from build123d import *

# Parameters (mm, degrees)
F1_DEPTH = 25.4
F2_W     = 190.5
F2_H     = 12.7
F2_W_2   = 19.05
F3_DEPTH = 254
F4_DEPTH = 25.4


with BuildPart() as f1:
    # F0 (on Top) → F1 (new body)
    with BuildSketch(Plane.XY):
        Polygon((170.6390685204, 0), (-165.9109314796, 0), (-165.9109314796, -161.925), (-153.2109314796, -161.925), (-153.2109314796, -25.4), (157.9390685204, -25.4), (157.9390685204, -161.925), (170.6390685204, -161.925), align=None)
    extrude(amount=F1_DEPTH)

    # F2 (on face) → F3 (join)
    with BuildSketch(Plane.XY.offset(25.4)):
        with Locations((2.3640685204, -19.05)):
            Rectangle(F2_W, F2_H)
        with Locations((2.3640685204, -6.35)):
            Rectangle(F2_W, F2_H)
        with Locations((-102.4109314796, -6.35)):
            Rectangle(F2_W_2, F2_H)
        with Locations((107.1390685204, -6.35)):
            Rectangle(F2_W_2, F2_H)
    extrude(amount=F3_DEPTH)

    # F2 (on face) → F4 (cut)
    with BuildSketch(Plane.XY.offset(25.4)):
        Polygon((116.6640685204, -12.7), (97.6140685204, -12.7), (97.6140685204, -25.4), (157.9390685204, -25.4), (157.9390685204, -12.7), align=None)
        Polygon((-92.8859314796, -25.4), (-92.8859314796, -12.7), (-111.9359314796, -12.7), (-153.2109314796, -12.7), (-153.2109314796, -25.4), align=None)
    extrude(amount=-F4_DEPTH, mode=Mode.SUBTRACT)


solid = f1.part
The model under review builds one solid part; all positions refer to its coordinate system, in mm. A direction names the side the tool comes from. Round coordinates to 2 decimals unless told otherwise and drop trailing zeros. Write each loop counter-clockwise with the first axis right and the second up, starting at its lowest first coordinate (ties: lowest second). Pieces come first, ordered by that corner, then holes. Notation, with made-up numbers: M -1,6.5 L 44,6.5 A25 cw 44,24.5 Z; hole C 20.25,16.25 d4. An arc over 180 degrees is marked long. Use a Markdown table: item, result. Add a question column.
Q1. We need section A-A, the plane y = -54. State the section outline as (x, z) points.
Q2. Machinability: for faces 4 (the face through (-111.936, -6, 151)), 5 (the face through (116.664, -6, 151)), 6 (the face through (115, -12.7, 111)), which of the approach directions +Z, -Z, +X, -X, +Y, -Y give a long, thin tool a straight path to every point of the face, cutting with its end or side? Answer none if there is none.
Q3. Insertion check: pin 1 (8 mm diameter, centred on x = 70.5, z = 106, fed in from -Y); pin 2 (10 mm diameter, centred on y = -5.5, z = 106, fed in from +X); pin 3 (6.5 mm diameter, centred on y = -9, z = 214.5, fed in from -X). Each pin has a flat end and moves straight along its axis. Give the tip position at first contact, or say it passes through.
Q4. The part is to be moulded in two halves that separate along X. For faces 1 (the face through (-165.911, -80, 13)), 2 (the face through (-160, -161.925, 13)), 3 (the face through (-110, -12.7, 107)), say which applies: pulls with the +X half, pulls with the -X half, needs draft (parallel to the pull), parting line crosses it, or undercut.
Q5. To check wall thickness, follow line 1 (Y direction, x = 94, z = 167); line 2 (X direction, y = -23, z = 193); line 3 (Y direction, x = 99.5, z = 183.5). State the ranges of each line that lie inside material, in increasing order.
Q6. We need section C-C, the plane x = -74. State the section outline as (y, z) points, plus the area to 3 significant figures.
Q7. We need section B-B, the plane z = 191.5. State the section outline as (x, y) points.
Findings below:
| question | item | result |
|---|---|---|
| 1 | outline | M -165.91,0 L -153.21,0 L -153.21,25.4 L -165.91,25.4 Z; M 157.94,0 L 170.64,0 L 170.64,25.4 L 157.94,25.4 Z |
| 2 | face 4 | +Z, -X, +Y, -Y |
| 2 | face 5 | +Z, +X, +Y, -Y |
| 2 | face 6 | +Z, -Z, -Y |
| 3 | pin 1 | stops at y = -25.4 |
| 3 | pin 2 | stops at x = 116.66 |
| 3 | pin 3 | stops at x = -111.94 |
| 4 | face 1 | pulls with the -X half |
| 4 | face 2 | needs draft |
| 4 | face 3 | undercut |
| 5 | line 1 | y = -25.4 to 0 |
| 5 | line 2 | x = -92.89 to 97.61 |
| 5 | line 3 | y = -12.7 to 0 |
| 6 | outline | M -25.4,0 L 0,0 L 0,279.4 L -25.4,279.4 Z |
| 6 | area | 7,100 mm² |
| 7 | outline | M -111.94,-12.7 L -92.89,-12.7 L -92.89,-25.4 L 97.61,-25.4 L 97.61,-12.7 L 116.66,-12.7 L 116.66,0 L -111.94,0 Z |
